```python
from build123d import *

# Parameters (mm, degrees)
SKETCH_2_W          = 22
SKETCH_2_H          = 40
EXTRUDE_1_DEPTH     = 4
SKETCH_3_W          = 22
SKETCH_3_H          = 2
EXTRUDE_2_DEPTH     = 10
SKETCH_4_R          = 1.5
CUT_EXTRUDE_1_DEPTH = 11
SKETCH_5_W          = 22
SKETCH_5_H          = 2
EXTRUDE_3_DEPTH     = 20
SKETCH_6_R          = 4
SKETCH_6_R_2        = 3
EXTRUDE_4_DEPTH     = 20
EXTRUDE_6_DEPTH     = 20


with BuildPart() as part:
    # Эскиз2 → Бобышка-Вытянуть1 (new body)
    with BuildSketch(Plane(origin=(0, 0, 0), x_dir=(1, 0, 0), z_dir=(0, 1, 0))):
        with Locations((-34.831985697, -10.44161698)):
            Rectangle(SKETCH_2_W, SKETCH_2_H)
    extrude(amount=EXTRUDE_1_DEPTH)

    # Эскиз3 → Бобышка-Вытянуть2 (add)
    with BuildSketch(Plane(origin=(0, 4, 0), x_dir=(1, 0, 0), z_dir=(0, 1, 0))):
        with Locations((-34.831985697, 8.55838302)):
            Rectangle(SKETCH_3_W, SKETCH_3_H)
        with Locations((-34.831985697, -0.44161698)):
            Rectangle(SKETCH_3_W, SKETCH_3_H)
    extrude(amount=EXTRUDE_2_DEPTH)

    # Эскиз4 → Вырез-Вытянуть1 (cut)
    with BuildSketch(Plane.XY.offset(1.44161698)):
        with Locations((-41.831985697, 9)):
            Circle(SKETCH_4_R)
        with Locations((-27.831985697, 9)):
            Circle(SKETCH_4_R)
    extrude(amount=-CUT_EXTRUDE_1_DEPTH, mode=Mode.SUBTRACT)

    # Эскиз5 → Бобышка-Вытянуть3 (add)
    with BuildSketch(Plane.XZ):
        with Locations((-34.831985697, 9.44161698)):
            Rectangle(SKETCH_5_W, SKETCH_5_H)
    extrude(amount=EXTRUDE_3_DEPTH)

    # Эскиз6 → Бобышка-Вытянуть4 (add)
    with BuildSketch(Plane.XY.offset(10.44161698)):
        with Locations(Location((-34.831985697, -10, 0), (0, 0, 180))):
            Circle(SKETCH_6_R)
        with Locations((-34.831985697, -10)):
            Circle(SKETCH_6_R_2, mode=Mode.SUBTRACT)
    extrude(amount=EXTRUDE_4_DEPTH)

    # Эскиз8 → Бобышка-Вытянуть6 (add)
    with BuildSketch(Plane.XZ):
        Polygon((-34.831985697, -8.063936519), (-28.331985697, 3.19439373), (-41.331985697, 3.19439373), align=None)
    extrude(amount=EXTRUDE_6_DEPTH)


solid = part.part
```
Verification items for the finished model (mm, model axes). A direction names the side the tool comes from. Coordinates: 2 decimals unless noted, no trailing zeros. Order: outer loops, then holes, each group sorted by start corner. A loop starts at its lowest first (then second) coordinate and runs counter-clockwise, first axis right, second up. Notation, with made-up numbers: (77.25, 70.5) -> (125.25, 70.5) arc R22 ccw to (125.25, 84.5) -> close; hole circle Ø2 at (43, 78.25). An arc over 180 degrees is marked (long way). Answer as CSV lines item,"result". Start each with the question number.
1) Cross-section at B-B, the plane y = -4.5. Record the boundary of the cut face in (x, z), then the cut area to 3 significant figures.
2) Set-up check for faces 4 (the face through (-35, -5, 10.442)), 5 (the face through (-35, -10, 3.194)), 6 (the face through (-35, 9, -7.558)), 7 (the face through (-35, 0, 20)), 8 (the face through (-31.627, -9.86, -2.514)): record each of +Z, -Z, +X, -X, +Y, -Y from which the full face is reachable in a straight line by a thin tool's end or side.
3) Release check for a two-part mould opening along Y. For faces 1 (the face through (-35, 4, 16)), 2 (the face through (-35, 2, 30.442)), 3 (the face through (-35, -10, 10.442)) record: released by +Y, released by -Y, zero draft, split by the parting line, or undercut.
4) Material ranges on L1, parallel to Y at x = -33.75, z = 13; L2, parallel to Z at x = -42.25, y = 5.5; L3, parallel to Y at x = -33.25, z = 18.5, recorded low to high. Write a range as [from, to].
5) Cross-section at C-C, the plane z = 11.5. Record the boundary of the cut face in (x, y), then the cut area to 3 significant figures.
6) Cross-section at D-D, the plane x = -44. Record the boundary of the cut face in (y, z), then the cut area to 3 significant figures.
7) Gauge pin test, flat ends, axial feed: pin 1 Ø2.5 at (x, y) = (-27.83, 9) entering from -Z; pin 2 Ø1.5 at (x, z) = (-37, 14) entering from +Y; pin 3 Ø5 at (x, y) = (-34, -9) entering from -Z; pin 4 Ø12 at (x, z) = (-33.5, 17) entering from -Y. Record the tip position at first contact, or that the pin passes through.
8) Cross-section at A-A, the plane y = 9. Record the boundary of the cut face in (x, z).
Conclusion:
1,outline,"(-45.83, 8.44) -> (-23.83, 8.44) -> (-23.83, 10.44) -> (-45.83, 10.44) -> close; (-41.33, 3.19) -> (-34.83, -8.06) -> (-28.33, 3.19) -> close"
1,area,"117 mm²"
2,face 4,"+Z"
2,face 5,"+X, -X, -Y"
2,face 6,"+X, -X, +Y"
2,face 7,"+Z, +X, -X"
2,face 8,"-Z, +X, -Y"
3,face 1,"released by +Y"
3,face 2,"zero draft"
3,face 3,"undercut"
4,L1,"y = [-13.85, -12.8], [-7.2, -6.15], [0, 4]"
4,L2,"z = [-9.56, -7.56], [-0.56, 1.44]"
4,L3,"y = [-13.67, -12.55], [-7.45, -6.33], [0, 4]"
5,outline,"(-45.83, 0) -> (-23.83, 0) -> (-23.83, 4) -> (-45.83, 4) -> close; circle Ø8 at (-34.83, -10); hole circle Ø6 at (-34.83, -10)"
5,area,"110 mm²"
6,outline,"(-20, 8.44) -> (0, 8.44) -> (0, -9.56) -> (14, -9.56) -> (14, -7.56) -> (4, -7.56) -> (4, -0.56) -> (14, -0.56) -> (14, 1.44) -> (4, 1.44) -> (4, 30.44) -> (0, 30.44) -> (0, 10.44) -> (-20, 10.44) -> close"
6,area,"240 mm²"
7,pin 1,"passes through"
7,pin 2,"stops at y = 4"
7,pin 3,"stops at z = -8.06"
7,pin 4,"stops at y = -14"
8,outline,"(-45.83, -9.56) -> (-43.33, -9.56) -> (-43.33, -7.56) -> (-45.83, -7.56) -> close; (-45.83, -0.56) -> (-43.33, -0.56) -> (-43.33, 1.44) -> (-45.83, 1.44) -> close; (-40.33, -9.56) -> (-29.33, -9.56) -> (-29.33, -7.56) -> (-40.33, -7.56) -> close; (-40.33, -0.56) -> (-29.33, -0.56) -> (-29.33, 1.44) -> (-40.33, 1.44) -> close; (-26.33, -9.56) -> (-23.83, -9.56) -> (-23.83, -7.56) -> (-26.33, -7.56) -> close; (-26.33, -0.56) -> (-23.83, -0.56) -> (-23.83, 1.44) -> (-26.33, 1.44) -> close"
